Could you check a few things on this model? Use its own coordinates, in mm. Face numbers are marked on the shaded views. A direction names the side the tool comes from. Round coordinates to 2 decimals unless told otherwise and drop trailing zeros. Order: outer loops, then holes, each group sorted by start corner. A loop starts at its lowest first (then second) coordinate and runs counter-clockwise, first axis right, second up.
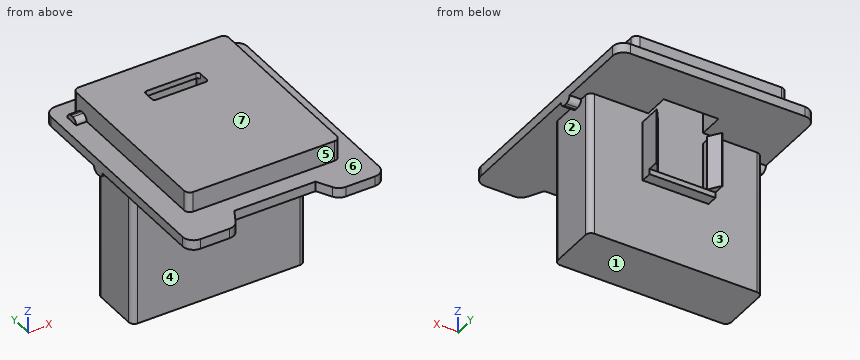
Autodesk Inventor part; units mm, degrees
ref_plane "YZ Plane" through (0, 0, 0) normal (1, 0, 0) x (0, 1, 0)
ref_plane "XZ Plane" through (0, 0, 0) normal (0, 1, 0) x (-1, 0, 0)
ref_plane "XY Plane" through (0, 0, 0) normal (0, 0, 1) x (1, 0, 0)
sketch "Sketch1" plane through (0, 0, 0) normal (0, 0, 1) x (1, 0, 0)
  line L0 (17.9, -19.1) -> (17.9, 19.1)
  line L1 (15.9, 21.1) -> (-15.9, 21.1)
  line L2 (-17.9, 19.1) -> (-17.9, -19.1)
  line L3 (-15.9, -21.1) -> (-10.5924, -21.1)
  line L4 (17.9, -21.1) -> (-17.9, 21.1) construction
  line L5 (17.9, 21.1) -> (-17.9, -21.1) construction
  line L6 (-7.4, -17.4) -> (7.4, -17.4)
  line L7 (-7.4, -17.4) -> (-8.833, -20.051)
  line L8 (7.4, -17.4) -> (8.833, -20.051)
  line L9 (10.5924, -21.1) -> (15.9, -21.1)
  line L10 (-9.4, -21.1) -> (9.4, -21.1)
  arc A0 (-15.9, 21.1) -> (-17.9, 19.1) centre (-15.9, 19.1) ccw
  arc A1 (17.9, 19.1) -> (15.9, 21.1) centre (15.9, 19.1) ccw
  arc A2 (15.9, -21.1) -> (17.9, -19.1) centre (15.9, -19.1) ccw
  arc A3 (8.833, -20.051) -> (10.5924, -21.1) centre (10.5924, -19.1) ccw
  arc A4 (-10.5924, -21.1) -> (-8.833, -20.051) centre (-10.5924, -19.1) ccw
  arc A5 (-17.9, -19.1) -> (-15.9, -21.1) centre (-15.9, -19.1) ccw
  point P0 (0, 0)
  dimension "d0" = 35.8
  dimension "d1" = 42.2
  dimension "d2" = 38.5
  dimension "d3" = 10.5
  dimension "d4" = 10.5
  dimension "d5" = 8.5
  dimension "d6" = 8.5
  dimension "d7" = 2
extrude "Extrusion1" add sketch "Sketch1" along normal blind 1.8
sketch "Sketch2" plane through (0, 0, 1.8) normal (0, 0, 1) x (1, 0, 0)
  line L0 (-15.85, 15.1) -> (15.85, 15.1)
  line L1 (15.85, 15.1) -> (15.85, 17.6)
  line L2 (15.85, 17.6) -> (-15.85, 17.6)
  line L3 (-15.85, 17.6) -> (-15.85, 15.1)
  line L4 (-15.85, 15.1) -> (15.85, 17.6) construction
  line L5 (15.85, 15.1) -> (-15.85, 17.6) construction
  line L6 (15.9, 21.1) -> (-15.9, 21.1)
  point P0 (0, 0)
  point P1 (0, 16.35)
  point P2 (0, 16.35)
  point P3 (15.85, 16.35)
  point P4 (-15.85, 16.35)
  dimension "d10" = 2.5
  dimension "d11" = 6
  dimension "d12" = 31.7
extrude "Extrusion2" add sketch "Sketch2" along normal blind 1
fillet "Fillet1" radius 1 2 edges at (0, 17.6, 2.8) (0, 15.1, 2.8)
sketch "Sketch3" plane through (0, 0, 1.8) normal (0, 0, 1) x (1, 0, 0)
  line L0 (-12.9, 19.1) -> (12.9, 19.1)
  line L1 (13.9, 18.1) -> (13.9, -13.2)
  line L2 (12.9, -14.2) -> (-12.9, -14.2)
  line L3 (-13.9, -13.2) -> (-13.9, 18.1)
  line L4 (15.9, 21.1) -> (-15.9, 21.1)
  line L5 (-13.9, 2.9131) -> (-17.9, 2.9131)
  line L6 (-17.9, 19.1) -> (-17.9, -19.1)
  line L7 (13.9, 2.9131) -> (17.9, 2.9131)
  line L8 (17.9, -19.1) -> (17.9, 19.1)
  arc A0 (-12.9, 19.1) -> (-13.9, 18.1) centre (-12.9, 18.1) ccw
  arc A1 (13.9, 18.1) -> (12.9, 19.1) centre (12.9, 18.1) ccw
  arc A2 (12.9, -14.2) -> (13.9, -13.2) centre (12.9, -13.2) ccw
  arc A3 (-13.9, -13.2) -> (-12.9, -14.2) centre (-12.9, -13.2) ccw
  point P0 (0, 0)
  point P1 (13.9, -14.2)
  point P2 (13.9, 19.1)
  point P3 (-13.9, -14.2)
  dimension "d16" = 27.8
  dimension "d17" = 33.3
  dimension "d18" = 2
  dimension "d19" = 1
extrude "Extrusion3" add sketch "Sketch3" along normal blind 3.7
sketch "Sketch4" plane through (0, 0, 0) normal (0, 0, -1) x (-1, 0, 0)
  line L0 (-17.9, -19.1) -> (-17.9, 19.1)
  line L1 (17.9, 19.1) -> (17.9, -19.1)
  line L2 (-17.9, 6.6) -> (17.9, 6.6)
  line L3 (17.9, 6.6) -> (17.9, 4.1)
  line L4 (17.9, 4.1) -> (-17.9, 4.1)
  line L5 (-17.9, 4.1) -> (-17.9, 6.6)
  line L6 (-15.9, 21.1) -> (15.9, 21.1)
  point P0 (0, 0)
  dimension "d22" = 2.5
  dimension "d23" = 17
extrude "Extrusion4" add sketch "Sketch4" along normal blind 1
fillet "Fillet2" radius 1 2 edges at (0, 6.6, -1) (0, 4.1, -1)
sketch "Sketch5" plane through (0, 0, 0) normal (0, 0, -1) x (-1, 0, 0)
  line L0 (-14.8, 8.9) -> (14.8, 8.9)
  line L1 (15.8, 7.9) -> (15.8, -0.1)
  line L2 (14.8, -1.1) -> (-14.8, -1.1)
  line L3 (-15.8, -0.1) -> (-15.8, 7.9)
  line L4 (-15.9, 21.1) -> (15.9, 21.1)
  line L5 (-17.9, 6.6) -> (-17.9, 19.1)
  line L6 (17.9, 4.1) -> (17.9, -19.1)
  arc A0 (-15.8, -0.1) -> (-14.8, -1.1) centre (-14.8, -0.1) ccw
  arc A1 (-14.8, 8.9) -> (-15.8, 7.9) centre (-14.8, 7.9) ccw
  arc A2 (15.8, 7.9) -> (14.8, 8.9) centre (14.8, 7.9) ccw
  arc A3 (14.8, -1.1) -> (15.8, -0.1) centre (14.8, -0.1) ccw
  point P0 (0, 0)
  point P1 (0, 8.9)
  dimension "d27" = 22.2
  dimension "d28" = 2.1
  dimension "d29" = 10
  dimension "d30" = 2.1
  dimension "d31" = 1
extrude "Extrusion5" add sketch "Sketch5" along normal blind 26.3
sketch "Sketch6" plane through (0, 0, 0) normal (0, 0, -1) x (-1, 0, 0)
  line L0 (-5, 13.4) -> (5, 13.4)
  line L1 (5, 13.4) -> (5, 8.9)
  line L2 (5, 8.9) -> (-5, 8.9)
  line L3 (-5, 8.9) -> (-5, 13.4)
  line L4 (14.8, 8.9) -> (-14.8, 8.9)
  line L5 (5, 13.4) -> (17.9, 13.4)
  line L6 (17.9, 19.1) -> (17.9, 6.6)
  line L7 (-5, 13.4) -> (-17.9, 13.4)
  line L8 (-17.9, -19.1) -> (-17.9, 19.1)
  point P0 (0, 0)
  point P1 (-5, 11.15)
  dimension "d34" = 10
  dimension "d60" = 4.5
extrude "Extrusion6" cut sketch "Sketch6" against normal blind 4.5
sketch "Sketch7" plane through (-14.8, 8.9, -26.3) normal (0, 1, 0) x (1, 0, 0)
  line L0 (9.8, -30.8) -> (19.8, -30.8)
  line L1 (14.8, -30.8) -> (14.8, -14.3)
  line L2 (8.8, -14.3) -> (20.8, -14.3)
  line L3 (20.8, -14.3) -> (20.8, -13.3)
  line L4 (20.8, -13.3) -> (8.8, -13.3)
  line L5 (8.8, -13.3) -> (8.8, -14.3)
  line L6 (20.8, -14.3) -> (20.8, -24.3)
  line L7 (20.8, -24.3) -> (19.8, -24.3)
  line L8 (19.8, -24.3) -> (19.8, -14.3)
  line L9 (8.8, -14.3) -> (8.8, -24.3)
  line L10 (8.8, -24.3) -> (9.8, -24.3)
  line L11 (9.8, -24.3) -> (9.8, -14.3)
  point P0 (14.8, -26.3)
  point P1 (20.3, -24.3)
  dimension "d38" = 12
  dimension "d39" = 1
  dimension "d40" = 1
  dimension "d58" = 16.5
  dimension "d59" = 10
extrude "Extrusion7" add sketch "Sketch7" along normal blind 2
sketch "Sketch8" plane through (-14.8, 10.9, -26.3) normal (0, 1, 0) x (1, 0, 0)
  line L0 (9.8, -14.3) -> (19.8, -14.3)
  line L1 (20.8, -24.3) -> (20.8, -13.3)
  line L2 (19.8, -14.3) -> (20.8, -14.3)
  line L3 (20.8, -14.3) -> (20.8, -24.3)
  line L4 (20.8, -24.3) -> (19.8, -24.3)
  line L5 (19.8, -24.3) -> (19.8, -14.3)
  line L6 (9.8, -14.3) -> (9.8, -30.8)
  line L7 (8.8, -24.3) -> (8.8, -13.3)
  line L8 (9.8, -14.3) -> (8.8, -14.3)
  line L9 (8.8, -14.3) -> (8.8, -24.3)
  line L10 (8.8, -24.3) -> (9.8, -24.3)
  line L11 (9.8, -24.3) -> (9.8, -14.3)
  point P0 (14.8, -26.3)
  point P1 (9.8, -24.3)
  point P2 (9.8, -24.3)
  point P3 (8.8, -14.3)
  point P4 (20.8, -26.3)
  point P5 (8.8, -26.3)
extrude "Extrusion8" add sketch "Sketch8" along normal blind 2
sketch "Sketch9" plane through (5, 8.9, -12) normal (-1, 0, 0) x (0, 0, 1)
  line L0 (0, 2) -> (0, 4)
  line L1 (10, 0) -> (10, 4)
  line L2 (0, 4) -> (10, 4)
  line L3 (10, 4) -> (10, 2)
  line L4 (10, 2) -> (0, 2)
  line L5 (0, 2) -> (0, 4)
  point P0 (12, -8.9)
extrude "Extrusion9" add sketch "Sketch9" along normal blind 0.5
chamfer "Chamfer1" distance 2 angle 35 1 edges at (4.5, 12.9, -7) measured on face at (4.5, 12.2333, -8.6667)
mirror "Mirror1" about plane through (0, 0, 0) normal (1, 0, 0) of "Extrusion9", "Chamfer1"
sketch "Sketch10" plane through (0, 0, 4.5) normal (0, 0, -1) x (-1, 0, 0)
  line L0 (-4.5, 9.9) -> (4.5, 9.9)
  line L1 (5, 10.4) -> (5, 12.2)
  line L2 (4.5, 12.7) -> (-4.5, 12.7)
  line L3 (-5, 12.2) -> (-5, 10.4)
  line L4 (5, 8.9) -> (-5, 8.9)
  line L5 (-5, 8.9) -> (-5, 13.4)
  arc A0 (-5, 10.4) -> (-4.5, 9.9) centre (-4.5, 10.4) ccw
  arc A1 (-4.5, 12.7) -> (-5, 12.2) centre (-4.5, 12.2) ccw
  arc A2 (5, 12.2) -> (4.5, 12.7) centre (4.5, 12.2) ccw
  arc A3 (4.5, 9.9) -> (5, 10.4) centre (4.5, 10.4) ccw
  point P0 (0, 0)
  point P1 (-5, 11.3)
  dimension "d51" = 1
  dimension "d52" = 10
  dimension "d53" = 0.5
  dimension "d54" = 2.8
extrude "Extrusion10" cut sketch "Sketch10" against normal blind 2
properties part number "PS2 USB C PD Mount"
Q1. Imagine slicing it at C-C, the plane x = 12. Please give me the cut outline in (y, z), then the cut area to 3 significant figures.
Q2. For the marked faces 4, 5, 6 and 7, which set-ups out of +Z, -Z, +X, -X, +Y, -Y let a thin tool reach every point of the face, with its end or its side?
Q3. Imagine slicing it at A-A, the plane x = -1. Please give me the cut outline in (y, z).
Q4. Imagine slicing it at B-B, the plane y = 14. Please give me the cut outline in (x, z).
Q5. For P1, Ø0.9, axis at x = -0.5, z = 0.5, coming from the -Y side; P2, Ø2, axis at y = 11.5, z = 3, coming from the -X side; P3, Ø8, axis at y = 12.5, z = -14, coming from the -X side; P4, Ø4, axis at x = -10.5, y = 9.5, coming from the -Z side, each with a flat end and sliding along its axis, tell me the tip position at first contact or that it passes through.
Q6. We'd pull the mould along X, two halves only. Please class the marked faces 1, 2 and 3: released by +X, released by -X, zero draft, split by the parting line, or undercut.
Q7. I need wall thicknesses on L1, parallel to X at y = 10.5, z = -9; L2, parallel to X at y = 13, z = 2.5; L3, parallel to Y at x = -6.5, z = -24. Which ranges of each line are inside material? Lowest first, please.
Filled in:
1. outline: (-21.1, 0) - (-1.1, 0) - (-1.1, -26.3) - (8.9, -26.3) - (8.9, 0) - (21.1, 0) - (21.1, 1.8) - (19.1, 1.8) - (19.1, 5.5) - (-14.2, 5.5) - (-14.2, 1.8) - (-21.1, 1.8) - close
1. area: 462 mm2
2. face 4: -Z, +X, -X, -Y
2. face 5: +Z, +X, -X, -Y
2. face 6: +Z
2. face 7: +Z, +X, -X, +Y, -Y
3. outline: (-17.4, 0) - (-1.1, 0) - (-1.1, -26.3) - (8.9, -26.3) - (8.9, -13) - (10.9, -13) - (10.9, -12) - (8.9, -12) - (8.9, 4.5) - (9.9, 4.5) - (9.9, 5.5) - (-14.2, 5.5) - (-14.2, 1.8) - (-17.4, 1.8) - close; (12.7, 4.5) - (13.4, 4.5) - (13.4, 0) - (21.1, 0) - (21.1, 1.8) - (19.1, 1.8) - (19.1, 5.5) - (12.7, 5.5) - close
4. outline: (-17.9, 0) - (17.9, 0) - (17.9, 1.8) - (13.9, 1.8) - (13.9, 5.5) - (-13.9, 5.5) - (-13.9, 1.8) - (-17.9, 1.8) - close
5. P1: stops at y = -17.4
5. P2: stops at x = -13.9
5. P3: stops at x = -15.6
5. P4: stops at z = -26.3
6. face 1: zero draft
6. face 2: released by +X
6. face 3: undercut
7. L1: x = -6 to -5, 5 to 6
7. L2: x = -13.9 to -5, 5 to 13.9
7. L3: y = -1.1 to 8.9
